Answer from the drawing. Dimensions are ordinates in mm from the lowest x, y and z of the part. Coordinates: 2 decimals unless noted, no trailing zeros. Write each loop counter-clockwise with the first axis right and the second up, starting at its lowest first coordinate (ties: lowest second). Pieces come first, ordered by that corner, then holes. Notation, with made-up numbers: (8, -30) - (31, -30) arc R14 cw to (31, -20) - close; hole circle Ø4 at (10, 15.25). An arc over 180 degrees is marked (long way). Return JSON: item names as keys, results as strings.
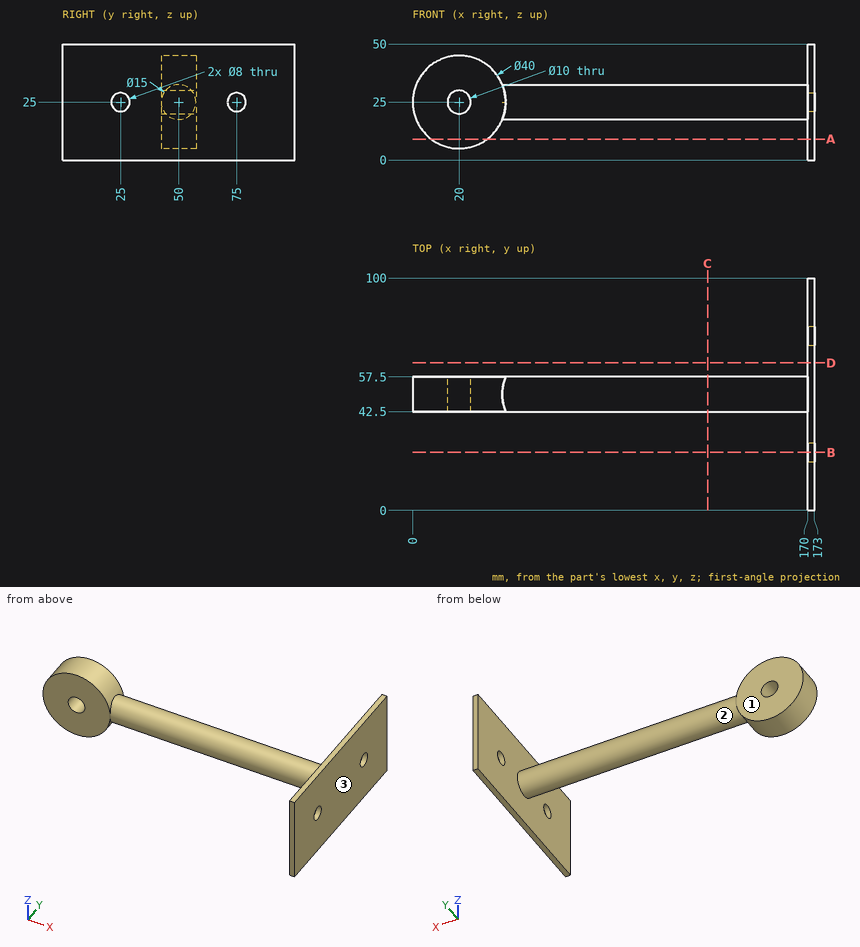
(1) A cutting plane is placed at D-D (y = 63.5). Determine the outline of the cut face in (x, z), and give its area (3 significant figures).
Answer:
{"outline": "(170, 0) - (173, 0) - (173, 50) - (170, 50) - close", "area": "150 mm²"}
(2) Determine the mould class of the marked faces 1, 2 and 3 for opening direction X: +X half, -X half, draft (parallel to the pull), parting line (faces both ways), or undercut.
Answer:
{"face 1": "draft", "face 2": "undercut", "face 3": "+X half"}
(3) A cutting plane is placed at C-C (x = 127). Determine the outline of the cut face in (y, z).
Answer:
{"outline": "circle Ø15 at (50, 25)"}
(4) A cutting plane is placed at A-A (z = 9). Determine the outline of the cut face in (x, y).
Answer:
{"outline": "(8, 42.5) - (32, 42.5) - (32, 57.5) - (8, 57.5) - close; (170, 0) - (173, 0) - (173, 100) - (170, 100) - close"}
(5) Flat-ended cylindrical pins translate along their axes: P1, Ø6, axis at x = 32.5, z = 19.5, coming from the -Y side; P2, Ø7, axis at y = 75, z = 25, coming from the -X side; P3, Ø2, axis at x = 130.5, y = 44, coming from the +Z side; P4, Ø13, axis at y = 25, z = 25, coming from the -X side. Find the tip coordinate at first contact, or state that the pin passes through.
Answer:
{"P1": "y = 42.5", "P2": "through", "P3": "z = 30.59", "P4": "x = 170"}
(6) A cutting plane is placed at B-B (y = 25). Determine the outline of the cut face in (x, z).
Answer:
{"outline": "(170, 0) - (173, 0) - (173, 21) - (170, 21) - close; (170, 29) - (173, 29) - (173, 50) - (170, 50) - close"}
(7) Straight lines are drawn through the part: line 1 (Z direction, x = 172.15, y = 75); line 2 (Y direction, x = 15, z = 19); line 3 (Z direction, x = 20, y = 54). For each, find the intervals that lie inside material, in ascending order. Write a range as from..to.
Answer:
{"line 1": "0..21, 29..50", "line 2": "42.5..57.5", "line 3": "5..20, 30..45"}
